Read the model definition and answer for the solid it produces. Units are mm, in the model's axes. Coordinates: 2 decimals unless noted, no trailing zeros. Write each loop counter-clockwise with the first axis right and the second up, starting at its lowest first coordinate (ties: lowest second). Pieces come first, ordered by that corner, then holes. Notation, with made-up numbers: (37, 43.5) -> (79, 43.5) arc R7 cw to (79, 47.5) -> close; hole circle Ø4 at (77, 18). An arc over 180 degrees is marked (long way). Write item = value, one per line. Start each with the question number.
1) Section A-A (y = 0.55) is taken. Count the separate pieces of the cut face and the enclosed holes in it, plus the area to 3 significant figures.
2) For a pull along Z with two mould halves and no side action, classify faces 1 (the face through (46.53, 1.52, -3.39)), 2 (the face through (25, 0, -5)), 3 (the face through (1, 2, -8)), 4 (the face through (3.338, 1.521, -3.616)) as released by +Z, released by -Z, zero draft, split by the parting line, or undercut.
3) Flat-ended cylindrical pins translate along their axes: pin 1 Ø1.5 at (x, z) = (15.5, -2) entering from -Y; pin 2 Ø1 at (y, z) = (2.5, -3.5) entering from -X. Find the tip coordinate at first contact, or state that the pin passes through.
4) Find the intervals of material crossed by line 1 along X through (y, z) = (0.85, -5); line 2 along X through (y, z) = (2.55, -2.5); line 3 along Z through (x, y) = (48.5, 2.4), in increasing order. Write a range as from..to.
5) Section C-C (x = 4) is taken. Determine the outline of the cut face in (y, z), plus the area to 3 significant figures.
6) Section B-B (x = 44) is taken. Determine the outline of the cut face in (y, z).
from build123d import *

# Parameters (mm, degrees)
SKETCH2_W           = 50
SKETCH2_H           = 10
BOSS_EXTRUDE1_DEPTH = 3
FILLET1_R           = 5
FILLET2_R           = 5
SKETCH9_R           = 3
CUT_EXTRUDE2_DEPTH  = 52.078371156
SKETCH10_R          = 3
CUT_EXTRUDE3_DEPTH  = 52.078371156


with BuildPart() as part:
    # Sketch2 → Boss-Extrude1 (new body)
    with BuildSketch(Plane(origin=(0, 0, 0), x_dir=(1, 0, 0), z_dir=(0, 1, 0))):
        with Locations((25, 5)):
            Rectangle(SKETCH2_W, SKETCH2_H)
    extrude(amount=BOSS_EXTRUDE1_DEPTH)

    # Fillet1
    fillet1_edges = [part.edges().sort_by_distance(p)[0] for p in [
        (0, 1.5, -10),
        (0, 1.5, 0),
    ]]
    fillet(fillet1_edges, radius=FILLET1_R - 0.0001)  # a hair under: the kernel refuses the full size

    # Fillet2
    fillet2_edges = [part.edges().sort_by_distance(p)[0] for p in [
        (50, 1.5, -10),
        (50, 1.5, 0),
    ]]
    fillet(fillet2_edges, radius=FILLET2_R - 0.0001)  # a hair under: the kernel refuses the full size

    # Sketch9 → Cut-Extrude2 (cut, through all)
    with BuildSketch(Plane(origin=(0, 3, 0), x_dir=(1, 0, 0), z_dir=(0, 1, 0))):
        with Locations(Location((6, 5, 0), (0, 0, 270))):
            Circle(SKETCH9_R)
    extrude(amount=-CUT_EXTRUDE2_DEPTH, mode=Mode.SUBTRACT)

    # Sketch10 → Cut-Extrude3 (cut, through all)
    with BuildSketch(Plane(origin=(0, 3, 0), x_dir=(1, 0, 0), z_dir=(0, 1, 0))):
        with Locations(Location((44, 5, 0), (0, 0, 270))):
            Circle(SKETCH10_R)
    extrude(amount=-CUT_EXTRUDE3_DEPTH, mode=Mode.SUBTRACT)


solid = part.part
Answer key:
q1.separate_pieces = 1
q1.enclosed_holes = 2
q1.area = 422 mm^2
q2.face_1 = undercut
q2.face_2 = zero draft
q2.face_3 = released by -Z
q2.face_4 = undercut
q3.pin_1 = 0
q3.pin_2 = 0.1
q4.line_1 = 0..3, 9..41, 47..50
q4.line_2 = 0.67..4.34, 7.66..42.34, 45.66..49.33
q4.line_3 = -8.57..-1.43
q5.outline = (0, -9.9) -> (3, -9.9) -> (3, -7.24) -> (0, -7.24) -> close; (0, -2.76) -> (3, -2.76) -> (3, -0.1) -> (0, -0.1) -> close
q5.area = 16.0 mm^2
q6.outline = (0, -10) -> (3, -10) -> (3, -8) -> (0, -8) -> close; (0, -2) -> (3, -2) -> (3, 0) -> (0, 0) -> close
